```python
from build123d import *

# Parameters (mm, degrees)
EXTRUDE_2_DEPTH     = 6
SKETCH_2_R          = 1.55
CUT_EXTRUDE_1_DEPTH = 10
SKETCH_3_R          = 1.55
CUT_EXTRUDE_2_DEPTH = 10
EXTRUDE_4_DEPTH     = 1.5
EXTRUDE_5_DEPTH     = 1.5
SKETCH_5_W          = 6
SKETCH_5_H          = 6
EXTRUDE_6_DEPTH     = 60
CUT_EXTRUDE_3_DEPTH = 60
SKETCH_9_W          = 6
SKETCH_9_H          = 8.845903007
EXTRUDE_7_DEPTH     = 60
SKETCH_11_R         = 1.55
CUT_EXTRUDE_5_DEPTH = 10
SKETCH_10_W         = 5
SKETCH_10_H         = 4
CUT_EXTRUDE_6_DEPTH = 10
EXTRUDE_8_DEPTH     = 2
EXTRUDE_9_DEPTH     = 2


with BuildPart() as part:
    # 草图1 → 凸台-拉伸2 (new body)
    with BuildSketch(Plane(origin=(0, 0, 0), x_dir=(1, 0, 0), z_dir=(0, 1, 0))):
        Polygon((-72.757575758, -68.484848485), (-72.757575758, -1.484848485), (71.242424242, -1.484848485), (71.242424242, -68.484848485), (74.242424242, -68.484848485), (74.242424242, -1.484848485), (74.242424242, 1.515151515), (71.242424242, 1.515151515), (-72.757575758, 1.515151515), (-75.757575758, 1.515151515), (-75.757575758, -1.484848485), (-75.757575758, -68.484848485), align=None)
    extrude(amount=EXTRUDE_2_DEPTH)

    # 草图2 → 切除-拉伸1 (cut)
    with BuildSketch(Plane(origin=(-72.757575758, 0, 0), x_dir=(0, 0, -1), z_dir=(1, 0, 0))):
        with Locations((-65.484848485, 3)):
            Circle(SKETCH_2_R)
    extrude(amount=-CUT_EXTRUDE_1_DEPTH, mode=Mode.SUBTRACT)

    # 草图3 → 切除-拉伸2 (cut)
    with BuildSketch(Plane(origin=(74.242424242, 0, 0), x_dir=(0, 0, -1), z_dir=(1, 0, 0))):
        with Locations((-65.484848485, 3)):
            Circle(SKETCH_3_R)
    extrude(amount=-CUT_EXTRUDE_2_DEPTH, mode=Mode.SUBTRACT)

    # 草图6 → 凸台-拉伸4 (add)
    with BuildSketch(Plane(origin=(0, 6, 0), x_dir=(1, 0, 0), z_dir=(0, 1, 0))):
        Polygon((-75.757575758, 1.515151515), (74.242424242, 1.515151515), (74.242424242, -68.484848485), (71.242424242, -68.484848485), (71.242424242, -1.484848485), (-72.757575758, -1.484848485), (-72.757575758, -68.484848485), (-75.757575758, -68.484848485), align=None)
    extrude(amount=EXTRUDE_4_DEPTH)

    # 草图7 → 凸台-拉伸5 (add)
    with BuildSketch(Plane.XZ):
        Polygon((-75.757575758, 68.484848485), (-75.757575758, -1.515151515), (74.242424242, -1.515151515), (74.242424242, 68.484848485), (71.242424242, 68.484848485), (71.242424242, 1.484848485), (-72.757575758, 1.484848485), (-72.757575758, 68.484848485), align=None)
    extrude(amount=EXTRUDE_5_DEPTH)

    # 草图5 → 凸台-拉伸6 (add)
    with BuildSketch(Plane(origin=(0, 0, -1.515151515), x_dir=(-1, 0, 0), z_dir=(0, 0, -1))):
        with Locations((0.757575758, 3)):
            Rectangle(SKETCH_5_W, SKETCH_5_H)
    extrude(amount=EXTRUDE_6_DEPTH)

    # 草图8 → 切除-拉伸3 (cut)
    with BuildSketch(Plane(origin=(2.242424242, 0, 0), x_dir=(0, 0, -1), z_dir=(1, 0, 0))):
        Polygon((61.515151515, 6), (55.015151515, 0), (61.515151515, 0), align=None)
    extrude(amount=-CUT_EXTRUDE_3_DEPTH, mode=Mode.SUBTRACT)

    # 草图9 → 凸台-拉伸7 (add)
    with BuildSketch(Plane(origin=(0, -27.419692129, -25.310485042), x_dir=(1, 0, 0), z_dir=(0, -0.7348034446274878, -0.678280102733066))):
        with Locations((-0.757575758, -44.848274344)):
            Rectangle(SKETCH_9_W, SKETCH_9_H)
    extrude(amount=EXTRUDE_7_DEPTH)

    # 草图11 → 切除-拉伸5 (cut)
    with BuildSketch(Plane(origin=(0, 33.419692129, -36.204666473), x_dir=(-1, 0, 0), z_dir=(0, 0.6782801027330662, -0.7348034446274876))):
        with Locations(Location((0.757575758, -90.315682622, 0), (0, 0, 90))):
            Circle(SKETCH_11_R)
    extrude(amount=-CUT_EXTRUDE_5_DEPTH, mode=Mode.SUBTRACT)

    # 草图10 → 切除-拉伸6 (cut)
    with BuildSketch(Plane(origin=(0, -71.507898807, -66.007291206), x_dir=(1, 0, 0), z_dir=(0, -0.7348034446274876, -0.6782801027330662))):
        with Locations((-0.757575758, -44.848274343)):
            Rectangle(SKETCH_10_W, SKETCH_10_H)
    extrude(amount=-CUT_EXTRUDE_6_DEPTH, mode=Mode.SUBTRACT)

    # 草图12 → 凸台-拉伸8 (add)
    with BuildSketch(Plane.ZY.offset(3.757575758)):
        Polygon((-102.211957679, -38.088206678), (-95.711957679, -44.088206678), (-55.015151515, 0), (-1.515151515, 0), (-1.515151515, 6), (-61.515151515, 6), align=None)
    extrude(amount=EXTRUDE_8_DEPTH)

    # 草图13 → 凸台-拉伸9 (add)
    with BuildSketch(Plane(origin=(2.242424242, 0, 0), x_dir=(0, 0, -1), z_dir=(1, 0, 0))):
        Polygon((95.711957679, -44.088206678), (102.211957679, -38.088206678), (61.515151515, 6), (1.515151515, 6), (1.515151515, 0), (55.015151515, 0), align=None)
    extrude(amount=EXTRUDE_9_DEPTH)


solid = part.part
```
Here's how the part is built. I have some questions about the finished solid (model axes, mm). A direction names the side the tool comes from. Coordinates: 2 decimals unless noted, no trailing zeros. Write each loop counter-clockwise with the first axis right and the second up, starting at its lowest first coordinate (ties: lowest second). Pieces come first, ordered by that corner, then holes. Notation, with made-up numbers: (76.25, -3.5) -> (132.25, -3.5) arc R13 ccw to (132.25, 10.5) -> close; hole circle Ø10 at (60.25, 47). An arc over 180 degrees is marked (long way). Use a Markdown table: item, result. Add a question column.
(1) If we section it at D-D, the plane x = 48: Write out the boundary of the cut face in (y, z), and give its area (3 significant figures).
(2) For faces 4 (the flat face through (71.242, 3, 35)), 5 (the flat face through (1.742, -37, -96)), 6 (the flat face through (-5.758, -8, -63)), 7 (the flat face through (-1, 0, -28)), 8 (the flat face through (-1, 6, -32)), which set-ups out of +Z, -Z, +X, -X, +Y, -Y let a thin tool reach every point of the face, with its end or its side?
(3) If we section it at A-A, the plane z = 54: Write out the boundary of the cut face in (x, y).
(4) If we section it at B-B, the plane y = -15: Write out the boundary of the cut face in (x, z), and give its area (3 significant figures).
(5) I'm going to push flat-ended pins straight in: P1, Ø8, axis at y = -37.5, z = -97, coming from the +X side; P2, Ø2, axis at x = 0, z = -84, coming from the -Y side; P3, Ø10, axis at x = -11, y = 4, coming from the -Z side; P4, Ø4, axis at y = 3, z = 65.48, coming from the -X side. Where does each tip first touch, or does it pass through?
(6) We'd pull the mould along X, two halves only. Please class faces 1 (the flat face through (74.242, 3, 33)), 2 (the flat face through (-34, -1.5, 0)), 3 (the cylindrical face through (-0.689, -39.249, -92.917)): +X half, -X half, draft (parallel to the pull), parting line (faces both ways), or undercut.
(7) Please list where these lines run through material, in increasing order: line 1 (X direction, y = -1, z = 4); line 2 (Z direction, x = -59, y = 4.5); line 3 (X direction, y = -3, z = -63.5).
(8) If we section it at C-C, the plane z = -69: Write out the boundary of the cut face in (x, y), and give its area (3 significant figures).
Outcome:
| question | item | result |
|---|---|---|
| 1 | outline | (-1.5, -1.52) -> (7.5, -1.52) -> (7.5, 1.48) -> (-1.5, 1.48) -> close |
| 1 | area | 27.0 mm^2 |
| 2 | face 4 | +Z, +Y, -Y |
| 2 | face 5 | none |
| 2 | face 6 | -Z, -X, +Y, -Y |
| 2 | face 7 | +X, -X, -Y |
| 2 | face 8 | -Z, +X, -X, +Y |
| 3 | outline | (-75.76, -1.5) -> (-72.76, -1.5) -> (-72.76, 7.5) -> (-75.76, 7.5) -> close; (71.24, -1.5) -> (74.24, -1.5) -> (74.24, 7.5) -> (71.24, 7.5) -> close |
| 4 | outline | (-5.76, -80.9) -> (4.24, -80.9) -> (4.24, -68.86) -> (-5.76, -68.86) -> close |
| 4 | area | 120 mm^2 |
| 5 | P1 | stops at x = 4.24 |
| 5 | P2 | stops at y = -32.48 |
| 5 | P3 | stops at z = -1.52 |
| 5 | P4 | stops at x = -75.76 |
| 6 | face 1 | +X half |
| 6 | face 2 | draft |
| 6 | face 3 | undercut |
| 7 | line 1 | x = -75.76 to -72.76, 71.24 to 74.24 |
| 7 | line 2 | z = -1.52 to 1.48 |
| 7 | line 3 | x = -5.76 to 4.24 |
| 8 | outline | (-5.76, -15.15) -> (4.24, -15.15) -> (4.24, -2.11) -> (-5.76, -2.11) -> close |
| 8 | area | 130 mm^2 |
